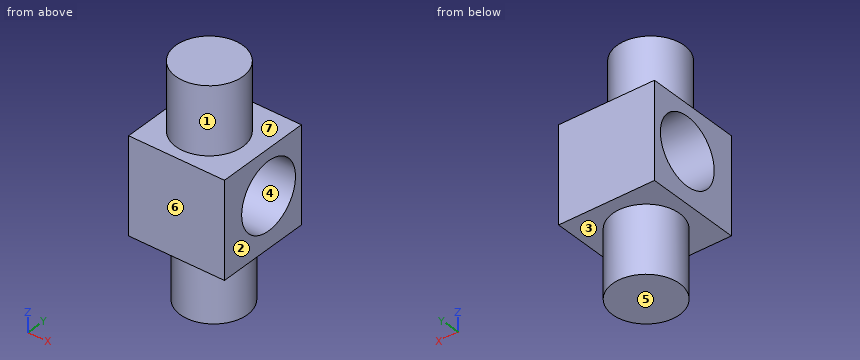
```python
from build123d import *

# Parameters (mm, degrees)
F0_W     = 100
F0_H     = 100
F1_DEPTH = 100
F2_R     = 35
F3_DEPTH = 70
F4_R     = 35
F5_DEPTH = 70
F7_D     = 70


with BuildPart() as f1:
    # F0 (on Front) → F1 (new body)
    with BuildSketch(Plane.XZ):
        with Locations((50, 50)):
            Rectangle(F0_W, F0_H)
    extrude(amount=F1_DEPTH)

    # F2 (on face) → F3 (join)
    with BuildSketch(Plane(origin=(0, 0, 0), x_dir=(1, 0, 0), z_dir=(0, 0, -1))):
        with Locations((48.01549, 49.015835)):
            Circle(F2_R)
    extrude(amount=F3_DEPTH)

    # F4 (on face) → F5 (join)
    with BuildSketch(Plane.XY.offset(100)):
        with Locations((47.09832, -53.716522)):
            Circle(F4_R)
    extrude(amount=F5_DEPTH)

    # F7 (through all)
    with Locations(Plane.YZ.offset(100)):
        with Locations((-42.680413, 52.683681)):
            Hole(F7_D / 2)


solid = f1.part
```
Can you work these out from the model? Positions are in its coordinate system, mm. Face numbers are marked on the shaded views. A direction names the side the tool comes from. Give positions to 0.01 mm unless a question says otherwise; leave off trailing zeros. Loops run counter-clockwise (first coordinate to the right, second up) from the corner with the lowest first, then second, coordinate; pieces in that order, holes last. Notation, with made-up numbers: M 49.25,4.5 L 94.25,4.5 A27 cw 94.25,42.5 Z; hole C 84,-1.75 d4. An arc over 180 degrees is marked long. Answer in a Markdown table with one row per item.
1. Which directions (+Z, -Z, +X, -X, +Y, -Y) give clear straight access to the entire face, cutting with the end or side of a thin tool? Please do the marked faces 1, 2 and 3.
Taken from the geometry:
| item | result |
|---|---|
| face 1 | +Z |
| face 2 | +Z, -Z, +X, +Y, -Y |
| face 3 | -Z |
2. Suppose I cut it at B-B on z = 44. Write out the boundary of the cut face in (x, y), plus the area to 3 significant figures.
Taken from the geometry:
| item | result |
|---|---|
| outline | M 0,-100 L 100,-100 L 100,-76.59 L 0,-76.59 Z; M 0,-8.77 L 100,-8.77 L 100,0 L 0,0 Z |
| area | 3,220 mm² |
3. Suppose I cut it at A-A on y = -35. Write out the boundary of the cut face in (x, z), plus the area to 3 significant figures.
Taken from the geometry:
| item | result |
|---|---|
| outline | M 0,0 L 15.94,0 L 15.94,-70 L 80.09,-70 L 80.09,0 L 100,0 L 100,18.54 L 0,18.54 Z; M 0,86.83 L 100,86.83 L 100,100 L 76.67,100 L 76.67,170 L 17.52,170 L 17.52,100 L 0,100 Z |
| area | 11,800 mm² |
4. Suppose I cut it at D-D on y = -71. Write out the boundary of the cut face in (x, z), plus the area to 3 significant figures.
Taken from the geometry:
| item | result |
|---|---|
| outline | M 0,0 L 20.78,0 L 20.78,-70 L 75.25,-70 L 75.25,0 L 100,0 L 100,32.12 L 0,32.12 Z; M 0,73.25 L 100,73.25 L 100,100 L 77.53,100 L 77.53,170 L 16.66,170 L 16.66,100 L 0,100 Z |
| area | 14,000 mm² |
5. Suppose I cut it at C-C on x = 88.5. Write out the boundary of the cut face in (y, z), plus the area to 3 significant figures.
Taken from the geometry:
| item | result |
|---|---|
| outline | M -100,0 L 0,0 L 0,100 L -100,100 Z; hole C -42.68,52.68 d70 |
| area | 6,150 mm² |
6. For pin 1 Ø1 at (x, y) = (80.5, -79) entering from +Z; pin 2 Ø3 at (x, z) = (35, 107) entering from +Y; pin 3 Ø12 at (x, z) = (75.5, 138) entering from -Y, each with a flat end and sliding along its axis, tell me the tip position at first contact or that it passes through.
Taken from the geometry:
| item | result |
|---|---|
| pin 1 | stops at z = 100 |
| pin 2 | stops at y = -20.36 |
| pin 3 | stops at y = -80.61 |
7. Thinking about a two-plate mould opening in Z: for the marked faces 4, 5, 6 and 7, which applies, released by +Z, released by -Z, zero draft, split by the parting line, or undercut?
Taken from the geometry:
| item | result |
|---|---|
| face 4 | undercut |
| face 5 | released by -Z |
| face 6 | zero draft |
| face 7 | released by +Z |
8. If I drill on line 1 along Z through (x, y) = (71.5, -51.5); line 2 along Z through (x, y) = (18, -66); line 3 along Y through (x, z) = (49, 26.5), over which ranges is the centre line in solid material (lowest first)?
Taken from the geometry:
| item | result |
|---|---|
| line 1 | z = -70 to 18.81, 86.55 to 170 |
| line 2 | z = -70 to 26.58, 78.78 to 170 |
| line 3 | y = -100 to -65.91, -19.46 to 0 |
